from build123d import *

# Parameters (mm, degrees)
ESQUISSE1_R             = 3.35
ESQUISSE1_R_2           = 2.85
BOSS_EXTRU_1_DEPTH      = 2
BOSS_EXTRU_2_DEPTH      = 14
ESQUISSE3_W             = 1.505412516
ESQUISSE3_H             = 3.452066632
BOSS_EXTRU_3_DEPTH      = 7
ENL_V_START             = -5
ESQUISSE4_R             = 2.85
ENL_V_MAT_EXTRU_1_DEPTH = 5


with BuildPart() as part:
    # Esquisse1 → Boss.-Extru.1 (new body)
    with BuildSketch(Plane.XY):
        Circle(ESQUISSE1_R)
        Circle(ESQUISSE1_R_2, mode=Mode.SUBTRACT)
    extrude(amount=BOSS_EXTRU_1_DEPTH)

    # Esquisse2 → Boss.-Extru.2 (add)
    with BuildSketch(Plane.XY.offset(2)):
        with BuildLine():
            Line((0, 3.35), (0, 2.85))
            ThreePointArc((0, 2.85), (-2.85, 0), (0, -2.85))
            Line((0, -2.85), (0, -3.35))
            ThreePointArc((0, -3.35), (-3.35, 0), (0, 3.35))
        make_face()
    extrude(amount=BOSS_EXTRU_2_DEPTH)

    # Esquisse3 → Boss.-Extru.3 (add)
    with BuildSketch(Plane(origin=(0, 0, 0), x_dir=(0, 0, -1), z_dir=(1, 0, 0))):
        with Locations((-14.566713218, 0)):
            Rectangle(ESQUISSE3_W, ESQUISSE3_H)
    extrude(amount=-BOSS_EXTRU_3_DEPTH)

    # Esquisse4 → Enlèv. mat.-Extru.1 (cut)
    with BuildSketch(Plane.XY.offset(16).offset(ENL_V_START)):
        with Locations(Location((0, 0, 0), (0, 0, 90))):
            Circle(ESQUISSE4_R)
    extrude(amount=ENL_V_MAT_EXTRU_1_DEPTH, mode=Mode.SUBTRACT)


solid = part.part
The model under review builds one solid part; all positions refer to its coordinate system, in mm. A direction names the side the tool comes from. Round coordinates to 2 decimals unless told otherwise and drop trailing zeros. Loops run counter-clockwise (first coordinate to the right, second up) from the corner with the lowest first, then second, coordinate; pieces in that order, holes last. Notation, with made-up numbers: M 39.25,-21.75 L 83.25,-21.75 A29 ccw 83.25,0.25 Z; hole C -38.5,-36 d5. An arc over 180 degrees is marked long. Answer as CSV lines item,"result". Start each with the question number.
Item 1: Consider section A-A (y = 0.25). Write out the cut boundary in (x, z).
Item 2: Mouldability with a two-part tool opening along Y and no side actions: class faces 3 (the face through (-2.847, 0.125, 7.888)), 4 (the face through (-5, 1.726, 15)), 5 (the face through (-5, -1.726, 15)), 6 (the face through (-5, 0, 13.814)) as released by +Y, released by -Y, zero draft, split by the parting line, or undercut.
Item 3: Consider section D-D (x = -4.5). Write out the cut boundary in (y, z).
Item 4: For faces 1 (the face through (-7, 0, 15)), 2 (the face through (3, 1, 2)), list the 3-axis set-ups (+Z, -Z, +X, -X, +Y, -Y) from which the entire face can be reached by the end or side of a thin tool; tool diameter is ignored.
Item 5: Wall thickness on line 1 (Z direction, x = -5.75, y = -0.25); line 2 (X direction, y = 0, z = 12); line 3 (Y direction, x = -2, z = 6.25): over which ranges is each line inside the solid? List them lowest first. Write a range as [from, to].
Item 6: Consider section B-B (x = 0.25). Write out the cut boundary in (y, z).
Item 7: Consider section C-C (y = -1.5). Write out the cut boundary in (x, z), then the cut area to 3 significant figures.
Item 8: Insertion check: P1, Ø1.5, axis at x = -5, z = 5.5, coming from the -Y side; P2, Ø0.5, axis at x = -5, z = 14.5, coming from the -Y side; P3, Ø0.6, axis at y = -3, z = 6.5, coming from the +X side; P4, Ø3.5, axis at x = 2, y = 0, coming from the +Z side. Each pin has a flat end and moves straight along its axis. Give the tip position at first contact, or say it passes through.
Answer:
1,outline,"M -7,13.81 L -3.34,13.81 L -3.34,0 L -2.84,0 L -2.84,16 L -3.34,16 L -3.34,15.32 L -7,15.32 Z; M 2.84,0 L 3.34,0 L 3.34,2 L 2.84,2 Z"
2,face 3,"undercut"
2,face 4,"released by +Y"
2,face 5,"released by -Y"
2,face 6,"zero draft"
3,outline,"M -1.73,13.81 L 1.73,13.81 L 1.73,15.32 L -1.73,15.32 Z"
4,face 1,"+Z, -Z, -X, +Y, -Y"
4,face 2,"+Z, +X, +Y, -Y"
5,line 1,"z = [13.81, 15.32]"
5,line 2,"x = [-3.35, -2.85]"
5,line 3,"y = [-2.69, -2.03], [2.03, 2.69]"
6,outline,"M -3.34,0 L -2.84,0 L -2.84,2 L -3.34,2 Z; M 2.84,0 L 3.34,0 L 3.34,2 L 2.84,2 Z"
7,outline,"M -7,13.81 L -3,13.81 L -3,0 L -2.42,0 L -2.42,16 L -3,16 L -3,15.32 L -7,15.32 Z; M 2.42,0 L 3,0 L 3,2 L 2.42,2 Z"
7,area,"16.3 mm^2"
8,P1,"passes through"
8,P2,"stops at y = -1.73"
8,P3,"stops at x = 0"
8,P4,"stops at z = 2"
